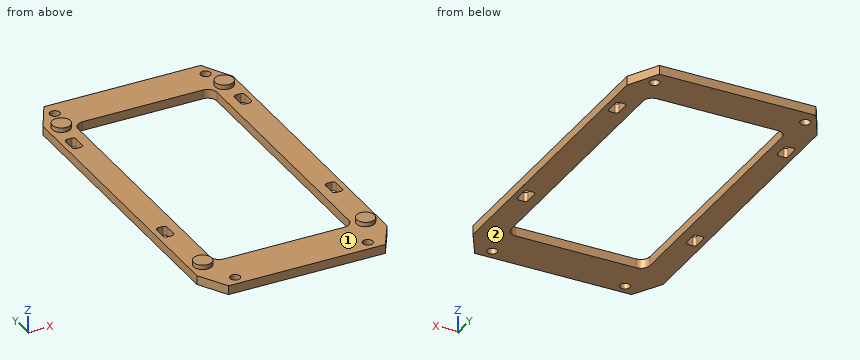
from build123d import *

# Parameters (mm, degrees)
SKETCH_4_R            = 1.65
EXTRUDE_258_DEPTH     = 3
CUT_EXTRUDE_383_DEPTH = 3
PCB_1P5MM_START       = 3
SKETCH_6_R            = 3
PCB_1P5MM_DEPTH       = 1.5


with BuildPart() as part:
    # 草图4 → Extrude 258 (new body)
    with BuildSketch(Plane.XY):
        Polygon((-26, -59.5), (26, -59.5), (31.5, -50), (31.5, 48), (26, 58), (-26, 58), (-31.5, 48), (-31.5, -50), align=None)
        with Locations((-22, -56)):
            Circle(SKETCH_4_R, mode=Mode.SUBTRACT)
        with Locations((-25, 53)):
            Circle(SKETCH_4_R, mode=Mode.SUBTRACT)
        with Locations((22, -56)):
            Circle(SKETCH_4_R, mode=Mode.SUBTRACT)
        with Locations((25, 53)):
            Circle(SKETCH_4_R, mode=Mode.SUBTRACT)
        with BuildLine():
            Line((-20, -45), (20, -45))
            ThreePointArc((20, -45), (22.121320344, -44.121320344), (23, -42))
            Line((23, -42), (23, 42))
            ThreePointArc((23, 42), (22.121320344, 44.121320344), (20, 45))
            Line((20, 45), (-20, 45))
            ThreePointArc((-20, 45), (-22.121320344, 44.121320344), (-23, 42))
            Line((-23, 42), (-23, -42))
            ThreePointArc((-23, -42), (-22.121320344, -44.121320344), (-20, -45))
        make_face(mode=Mode.SUBTRACT)
    extrude(amount=EXTRUDE_258_DEPTH)

    # 草图5 → Cut-Extrude 383 (cut)
    with BuildSketch(Plane.XY):
        with BuildLine():
            Line((-28.75, -26), (-27.25, -26))
            ThreePointArc((-27.25, -26), (-26.542893219, -25.707106781), (-26.25, -25))
            Line((-26.25, -25), (-26.25, -21))
            ThreePointArc((-26.25, -21), (-26.542893219, -20.292893219), (-27.25, -20))
            Line((-27.25, -20), (-28.75, -20))
            ThreePointArc((-28.75, -20), (-29.457106781, -20.292893219), (-29.75, -21))
            Line((-29.75, -21), (-29.75, -25))
            ThreePointArc((-29.75, -25), (-29.457106781, -25.707106781), (-28.75, -26))
        make_face()
        with BuildLine():
            Line((-28.75, 32), (-27.25, 32))
            ThreePointArc((-27.25, 32), (-26.542893219, 32.292893219), (-26.25, 33))
            Line((-26.25, 33), (-26.25, 37))
            ThreePointArc((-26.25, 37), (-26.542893219, 37.707106781), (-27.25, 38))
            Line((-27.25, 38), (-28.75, 38))
            ThreePointArc((-28.75, 38), (-29.457106781, 37.707106781), (-29.75, 37))
            Line((-29.75, 37), (-29.75, 33))
            ThreePointArc((-29.75, 33), (-29.457106781, 32.292893219), (-28.75, 32))
        make_face()
        with BuildLine():
            Line((27.25, -26), (28.75, -26))
            ThreePointArc((28.75, -26), (29.457106781, -25.707106781), (29.75, -25))
            Line((29.75, -25), (29.75, -21))
            ThreePointArc((29.75, -21), (29.457106781, -20.292893219), (28.75, -20))
            Line((28.75, -20), (27.25, -20))
            ThreePointArc((27.25, -20), (26.542893219, -20.292893219), (26.25, -21))
            Line((26.25, -21), (26.25, -25))
            ThreePointArc((26.25, -25), (26.542893219, -25.707106781), (27.25, -26))
        make_face()
        with BuildLine():
            Line((27.25, 32), (28.75, 32))
            ThreePointArc((28.75, 32), (29.457106781, 32.292893219), (29.75, 33))
            Line((29.75, 33), (29.75, 37))
            ThreePointArc((29.75, 37), (29.457106781, 37.707106781), (28.75, 38))
            Line((28.75, 38), (27.25, 38))
            ThreePointArc((27.25, 38), (26.542893219, 37.707106781), (26.25, 37))
            Line((26.25, 37), (26.25, 33))
            ThreePointArc((26.25, 33), (26.542893219, 32.292893219), (27.25, 32))
        make_face()
    extrude(amount=CUT_EXTRUDE_383_DEPTH, mode=Mode.SUBTRACT)

    # 草图6 → PCB下1p5mm绝缘支垫 (add)
    with BuildSketch(Plane.XY.offset(PCB_1P5MM_START)):
        with Locations((-27, -45)):
            Circle(SKETCH_6_R)
        with Locations((-27, 45)):
            Circle(SKETCH_6_R)
        with Locations((27, -45)):
            Circle(SKETCH_6_R)
        with Locations((27, 45)):
            Circle(SKETCH_6_R)
    extrude(amount=PCB_1P5MM_DEPTH)


solid = part.part
Source: CAD feature listing. Evaluate the final solid. Frame: model axes, mm. Face numbers are marked on the shaded views. Give positions to 0.01 mm unless a question says otherwise; leave off trailing zeros. Write each loop counter-clockwise with the first axis right and the second up, starting at its lowest first coordinate (ties: lowest second). Pieces come first, ordered by that corner, then holes. Notation, with made-up numbers: (-31.75, 32.25) -> (26.25, 32.25) arc R15 cw to (26.25, 51.25) -> close; hole circle Ø3 at (26.25, 4.5). An arc over 180 degrees is marked (long way). Return JSON: item names as keys, results as strings. Group by question number.
1. Pin query (flat end, axial travel): pin 1 Ø3 at (x, y) = (25, 53) entering from -Z; pin 2 Ø0.8 at (x, z) = (28, 1) entering from +Y; pin 3 Ø1.2 at (x, z) = (27.5, 1.5) entering from -Y; pin 4 Ø5.5 at (x, y) = (22, -56) entering from +Z. Return the tip coordinate at first contact, or that it passes through.
2. Material intervals for line 1 (X direction, y = 8, z = 2.4); line 2 (X direction, y = -21.5, z = 1.15); line 3 (Y direction, x = -17, z = 2.3), sorted ascending. Write a range as from..to.
3. Section A-A, the plane x = -0.5. Output: boundary loops of the cut face in (y, z), then the cut area to 3 significant figures.
4. Section D-D, the plane z = 1.1. Count the separate pieces of the cut face and the enclosed holes in it, then the cut area to 3 significant figures.
5. Mould query, pull axis Y, two halves, no side actions, for the marked faces 1 and 2. Classes: +Y half, -Y half, draft (parallel to the pull), parting line (faces both ways), or undercut.
6. Section B-B, the plane y = 2.5. Output: boundary loops of the cut face in (x, z), then the cut area to 3 significant figures.
7. Section C-C, the plane y = 53. Output: boundary loops of the cut face in (x, z).
Determined:
{
 "1": {"pin 1": "passes through", "pin 2": "stops at y = 55.09", "pin 3": "stops at y = -57.95", "pin 4": "stops at z = 3"},
 "2": {"line 1": "x = -31.5..-23, 23..31.5", "line 2": "x = -31.5..-29.75, -26.25..-23, 23..26.25, 29.75..31.5", "line 3": "y = -59.5..-45, 45..58"},
 "3": {"outline": "(-59.5, 0) -> (-45, 0) -> (-45, 3) -> (-59.5, 3) -> close; (45, 0) -> (58, 0) -> (58, 3) -> (45, 3) -> close", "area": "82.5 mm2"},
 "4": {"separate pieces": "1", "enclosed holes": "9", "area": "3,050 mm2"},
 "5": {"face 1": "undercut", "face 2": "draft"},
 "6": {"outline": "(-31.5, 0) -> (-23, 0) -> (-23, 3) -> (-31.5, 3) -> close; (23, 0) -> (31.5, 0) -> (31.5, 3) -> (23, 3) -> close", "area": "51.0 mm2"},
 "7": {"outline": "(-28.75, 0) -> (-26.65, 0) -> (-26.65, 3) -> (-28.75, 3) -> close; (-23.35, 0) -> (23.35, 0) -> (23.35, 3) -> (-23.35, 3) -> close; (26.65, 0) -> (28.75, 0) -> (28.75, 3) -> (26.65, 3) -> close"}
}
